Could you check a few things on this model? Use its own coordinates, in mm. A direction names the side the tool comes from. Give positions to 0.01 mm unless a question says otherwise; leave off trailing zeros. Write each loop counter-clockwise with the first axis right and the second up, starting at its lowest first coordinate (ties: lowest second). Pieces come first, ordered by that corner, then holes. Notation, with made-up numbers: (22.5, 59.25) - (33.5, 59.25) arc R20 ccw to (33.5, 78.25) - close; hole circle Ø8 at (43, -7.75). An arc over 180 degrees is marked (long way). Answer in a Markdown table with one row per item.
from build123d import *

# Parameters (mm, degrees)
SKETCH1_W            = 69.85
SKETCH1_H            = 38.1
SKETCH1_R            = 6.5
SKETCH1_R_2          = 8.5
BOSS_EXTRUDE1_DEPTH  = 5.8
M3_CLEARANCE_HOLE1_D = 3.4
CUT_EXTRUDE1_DEPTH   = 80.776390618
FILLET1_R            = 9.525


with BuildPart() as part:
    # Sketch1 → Boss-Extrude1 (new body)
    with BuildSketch(Plane.XY):
        with Locations((34.925, 19.05)):
            Rectangle(SKETCH1_W, SKETCH1_H)
        with Locations((58.939787697, 25.4)):
            Circle(SKETCH1_R, mode=Mode.SUBTRACT)
        with Locations((19.05, 25.4)):
            Circle(SKETCH1_R_2, mode=Mode.SUBTRACT)
    extrude(amount=BOSS_EXTRUDE1_DEPTH)

    # M3 Clearance Hole1 (through all)
    with Locations(Plane.XY.offset(5.8)):
        with Locations((30.05, 25.4), (24.55, 34.926279442), (13.55, 34.926279442), (8.05, 25.4), (13.55, 15.873720558), (24.55, 15.873720558)):
            Hole(M3_CLEARANCE_HOLE1_D / 2)

    # Sketch3 → Cut-Extrude1 (cut, through all)
    with BuildSketch(Plane.XY.offset(5.8)):
        with BuildLine():
            Line((31.75, 15.875), (31.75, 6.35))
            ThreePointArc((31.75, 6.35), (34.925, 3.175), (38.1, 6.35))
            Line((38.1, 6.35), (38.1, 15.875))
            ThreePointArc((38.1, 15.875), (34.925, 19.05), (31.75, 15.875))
        make_face()
    extrude(amount=-CUT_EXTRUDE1_DEPTH, mode=Mode.SUBTRACT)

    # Fillet1
    fillet1_edges = [part.edges().sort_by_distance(p)[0] for p in [
        (0, 0, 2.9),
        (0, 38.1, 2.9),
        (69.85, 38.1, 2.9),
        (69.85, 0, 2.9),
    ]]
    fillet(fillet1_edges, radius=FILLET1_R)


solid = part.part
1) Imagine slicing it at C-C (y = 29.5). List the corners of the cut face in (x, z) for me, then the cut area to 3 significant figures.
Check values:
| item | result |
|---|---|
| outline | (0.05, 0) - (11.6, 0) - (11.6, 5.8) - (0.05, 5.8) - close; (26.5, 0) - (53.9, 0) - (53.9, 5.8) - (26.5, 5.8) - close; (63.98, 0) - (69.8, 0) - (69.8, 5.8) - (63.98, 5.8) - close |
| area | 260 mm2 |
2) On a 3-axis mill with a long thin cutter (end or side, diameter ignored), from which of +Z, -Z, +X, -X, +Y, -Y can I reach the whole of each face in a straight line? I mean faces 4 (the face through (66.99, 35.38, 2.94)), 5 (the face through (31.75, 11, 3)). Say none if no direction works.
Check values:
| item | result |
|---|---|
| face 4 | +Z, -Z, +X, +Y |
| face 5 | +Z, -Z |
3) Imagine slicing it at A-A (x = 30.05). List the corners of the cut face in (y, z) for me, then the cut area to 3 significant figures.
Check values:
| item | result |
|---|---|
| outline | (0, 0) - (23.7, 0) - (23.7, 5.8) - (0, 5.8) - close; (27.1, 0) - (38.1, 0) - (38.1, 5.8) - (27.1, 5.8) - close |
| area | 201 mm2 |
4) If I drill on line 1 (X direction, y = 16, z = 4.1); line 2 (X direction, y = 12, z = 5.45); line 3 (X direction, y = 30.5, z = 1.75), over which ranges is the centre line in solid material (lowest first)?
Check values:
| item | result |
|---|---|
| line 1 | x = 0 to 11.85, 15.25 to 22.85, 26.25 to 31.75, 38.1 to 69.85 |
| line 2 | x = 0 to 31.75, 38.1 to 69.85 |
| line 3 | x = 0.2 to 12.25, 25.85 to 54.91, 62.97 to 69.65 |
5) We'd pull the mould along X, two halves only. Please class faces 1 (the face through (2.72, 35.24, 2.94)), 2 (the face through (35, 0, 3)), 3 (the face through (34.855, 3.176, 2.941)): +X half, -X half, draft (parallel to the pull), parting line (faces both ways), or undercut.
Check values:
| item | result |
|---|---|
| face 1 | -X half |
| face 2 | draft |
| face 3 | undercut |
6) Imagine slicing it at D-D (z = 3.9). State how many separate pieces and enclosed holes the cut face has, then the cut area to 3 significant figures.
Check values:
| item | result |
|---|---|
| separate pieces | 1 |
| enclosed holes | 9 |
| area | 2,080 mm2 |
7) Imagine slicing it at B-B (y = 25.4). List the corners of the cut face in (x, z) for me.
Check values:
| item | result |
|---|---|
| outline | (0, 0) - (6.35, 0) - (6.35, 5.8) - (0, 5.8) - close; (9.75, 0) - (10.55, 0) - (10.55, 5.8) - (9.75, 5.8) - close; (27.55, 0) - (28.35, 0) - (28.35, 5.8) - (27.55, 5.8) - close; (31.75, 0) - (52.44, 0) - (52.44, 5.8) - (31.75, 5.8) - close; (65.44, 0) - (69.85, 0) - (69.85, 5.8) - (65.44, 5.8) - close |
8) Will these pins go through, and if not, where does the flat tip stop? P1, Ø3, axis at x = 8.05, y = 25.4, coming from the +Z side; P2, Ø1, axis at y = 6.5, z = 4.5, coming from the +X side.
Check values:
| item | result |
|---|---|
| P1 | passes through |
| P2 | stops at x = 69.51 |
